Verification items for this drawing (mm, ordinates from the low corner). A direction names the side the tool comes from. Coordinates: 2 decimals unless noted, no trailing zeros. Order: outer loops, then holes, each group sorted by start corner. A loop starts at its lowest first (then second) coordinate and runs counter-clockwise, first axis right, second up. Notation, with made-up numbers: (-32, 73.25) -> (9, 73.25) arc R13 cw to (9, 84.25) -> close; hole circle Ø5 at (75.5, 42). An arc over 180 degrees is marked (long way). Answer in a Markdown table with one row per item. Add a question column.
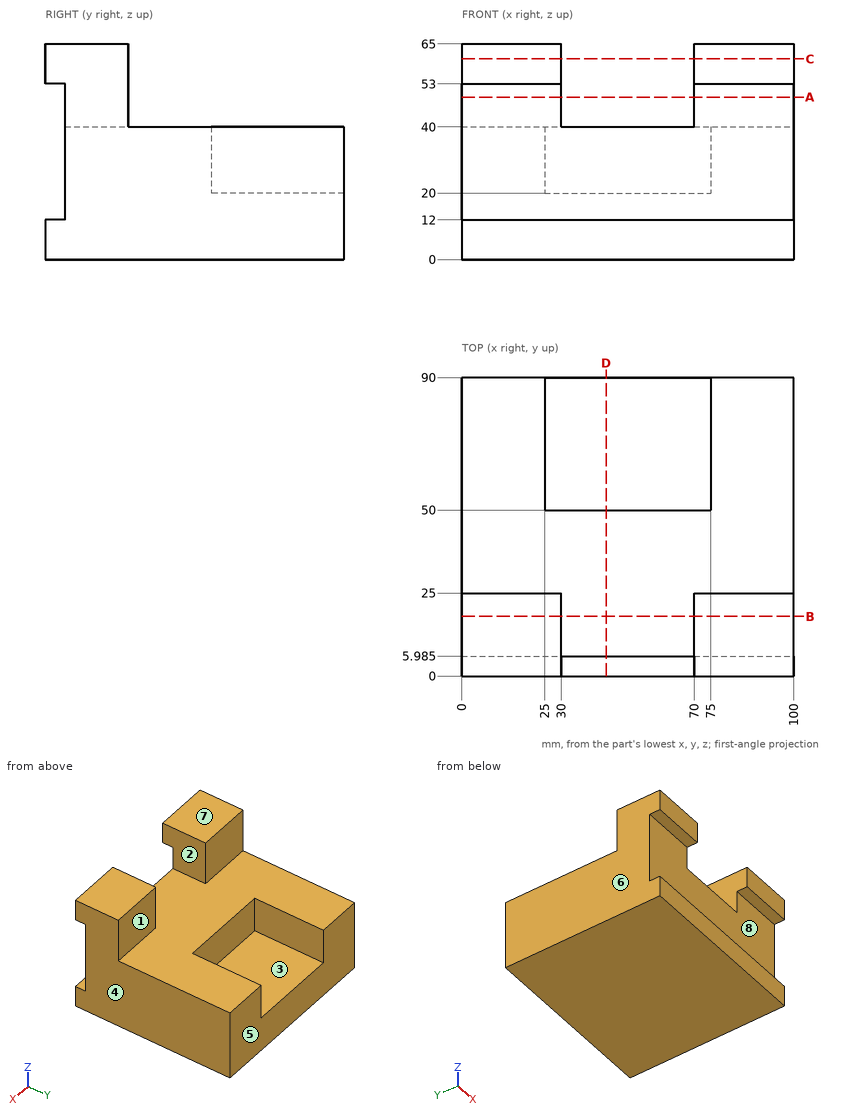
(1) Cross-section at A-A (z = 49). Enter the section's corners in (x, y) (3 decimals), plus the area to 3 significant figures.
(2) Go/stop test with flat-tipped pins: P1, Ø20, axis at x = 44, y = 74.5, coming from the +Z side; P2, Ø5, axis at x = 85, y = 73.5, coming from the +Z side; P3, Ø20, axis at x = 86.5, z = 58, coming from the +Y side. Record where each tip stops, or that it passes through.
(3) Cross-section at D-D (x = 43.5). Enter the section's corners in (y, z) (3 decimals), plus the area to 3 significant figures.
(4) Cross-section at B-B (y = 18). Enter the section's corners in (x, z), plus the area to 3 significant figures.
(5) Scan lines: line 1 along X through (y, z) = (10, 57); line 2 along Z through (x, y) = (92, 5.5); line 3 along X through (y, z) = (54, 34.5). Record each from-to range of solid material in increasing order.
(6) Mould release check, pull along Z, two halves, no side actions. Record for the marked faces 6, 7 and 8: +Z half, -Z half, draft (parallel to the pull), parting line (faces both ways), or undercut.
(7) Access from +Z, -Z, +X, -X, +Y, -Y to the whole of each face (thin tool, end or side, straight path). Record for the marked faces 1, 2, 3, 4 and 5.
(8) Cross-section at C-C (z = 60.5). Enter the section's corners in (x, y), plus the area to 3 significant figures.
Checks:
| question | item | result |
|---|---|---|
| 1 | outline | (0, 5.985) -> (30, 5.985) -> (30, 25) -> (0, 25) -> close; (70, 5.985) -> (100, 5.985) -> (100, 25) -> (70, 25) -> close |
| 1 | area | 1,140 mm² |
| 2 | P1 | z = 20 |
| 2 | P2 | z = 40 |
| 2 | P3 | y = 25 |
| 3 | outline | (0, 0) -> (90, 0) -> (90, 20) -> (50, 20) -> (50, 40) -> (5.985, 40) -> (5.985, 12) -> (0, 12) -> close |
| 3 | area | 2,630 mm² |
| 4 | outline | (0, 0) -> (100, 0) -> (100, 65) -> (70, 65) -> (70, 40) -> (30, 40) -> (30, 65) -> (0, 65) -> close |
| 4 | area | 5,500 mm² |
| 5 | line 1 | 0 to 30, 70 to 100 |
| 5 | line 2 | 0 to 12, 53 to 65 |
| 5 | line 3 | 0 to 25, 75 to 100 |
| 6 | face 6 | draft |
| 6 | face 7 | +Z half |
| 6 | face 8 | undercut |
| 7 | face 1 | +Z, +X, -X, +Y |
| 7 | face 2 | +Z, +Y, -Y |
| 7 | face 3 | +Z, +Y |
| 7 | face 4 | +Z, -Z, +X, +Y, -Y |
| 7 | face 5 | +Z, -Z, +X, -X, +Y |
| 8 | outline | (0, 0) -> (30, 0) -> (30, 25) -> (0, 25) -> close; (70, 0) -> (100, 0) -> (100, 25) -> (70, 25) -> close |
| 8 | area | 1,500 mm² |
